The model under review builds one solid part; all positions refer to its coordinate system, in mm. A direction names the side the tool comes from. Give positions to 0.01 mm unless a question says otherwise; leave off trailing zeros. Loops run counter-clockwise (first coordinate to the right, second up) from the corner with the lowest first, then second, coordinate; pieces in that order, holes last. Notation, with made-up numbers: M -23,34.25 L 12,34.25 A17 ccw 12,54.25 Z; hole C 28,-20.5 d5. An arc over 180 degrees is marked long. One line per item, written item: value. Start each with the question number.
Q1. For pin 1 (1.7 mm diameter, centred on x = -19, z = 5, fed in from +Y); pin 2 (12 mm diameter, centred on x = 0, y = 0, fed in from -Z); pin 3 (0.8 mm diameter, centred on x = -19, z = 7.5, fed in from +Y); pin 4 (5 mm diameter, centred on x = 0, y = 0, fed in from +Z), all flat-tipped, find the tip position at first contact; note any pin that passes through.
Q2. We need section A-A on z = 5. Give the number of separate pieces and of enclosed holes in the cut face, plus the area to 3 significant figures.
Q3. Mouldability with a two-part tool opening along Y and no side actions: class faces 6 (the face through (-15, 19, 10)), 7 (the face through (-23.4, 23.43, -2.46)), 8 (the face through (14.6, -9.05, 4.93)), 9 (the face through (-19, 16, 5)) as released by +Y, released by -Y, zero draft, split by the parting line, or undercut.
Q4. We need section B-B on x = 0. Write out the cut boundary in (y, z), plus the area to 3 significant figures.
Q5. We need section D-D on z = -2.25. Write out the cut boundary in (x, y), plus the area to 3 significant figures.
Q6. For faces 1 (the face through (14, -19, 10)), 2 (the face through (19, 13, 5)), 3 (the face through (14.6, 19.95, 4.93)), 4 (the face through (23.4, -23.43, -2.46)), 5 (the face through (14.43, -10.55, 4.93)), list the 3-axis set-ups (+Z, -Z, +X, -X, +Y, -Y) from which the entire face can be reached by the end or side of a thin tool; tool diameter is ignored.
Q7. To check wall thickness, follow line 1 along Y through (x, z) = (-13, 1.25); line 2 along X through (y, z) = (18, 2); line 3 along Y through (x, z) = (13.5, 7.5). State the ranges of each line that lie inside material, in increasing order. Write a range as from..to.
```python
from build123d import *

# Parameters (mm, degrees)
F0_W           = 36
F0_H           = 36
F1_DEPTH       = 4
F3_DEPTH       = 10
F5_D           = 8
F5_CSINK_D     = 15
F5_CSINK_ANGLE = 90
F6_DEPTH       = 1


with BuildPart() as f1:
    # F0 (on Top) → F1 (new body)
    with BuildSketch(Plane.XY):
        with BuildLine():
            ThreePointArc((24, 22), (23.4142135624, 23.4142135624), (22, 24))
            Line((22, 24), (-22, 24))
            ThreePointArc((-22, 24), (-23.4142135624, 23.4142135624), (-24, 22))
            Line((-24, 22), (-24, -22))
            ThreePointArc((-24, -22), (-23.4142135624, -23.4142135624), (-22, -24))
            Line((-22, -24), (22, -24))
            ThreePointArc((22, -24), (23.4142135624, -23.4142135624), (24, -22))
            Line((24, -22), (24, 22))
        make_face()
        Rectangle(F0_W, F0_H, mode=Mode.SUBTRACT)
        Rectangle(F0_W, F0_H)
    extrude(amount=-F1_DEPTH)

    # F2 (on face) → F3 (join)
    with BuildSketch(Plane.XY):
        with BuildLine():
            Line((18.1541072781, 16), (19.7395133362, 16))
            ThreePointArc((19.7395133362, 16), (14.5, 19.95), (9.2604866638, 16))
            Line((9.2604866638, 16), (10.8458927219, 16))
            ThreePointArc((10.8458927219, 16), (14.5, 18.45), (18.1541072781, 16))
        make_face()
        with BuildLine():
            ThreePointArc((9.2604866638, 13), (14.5, 9.05), (19.7395133362, 13))
            Line((19.7395133362, 13), (18.1541072781, 13))
            ThreePointArc((18.1541072781, 13), (14.5, 10.55), (10.8458927219, 13))
            Line((10.8458927219, 13), (9.2604866638, 13))
        make_face()
        with BuildLine():
            Line((-10.8458927219, 16), (-9.2604866638, 16))
            ThreePointArc((-9.2604866638, 16), (-14.5, 19.95), (-19.7395133362, 16))
            Line((-19.7395133362, 16), (-18.1541072781, 16))
            ThreePointArc((-18.1541072781, 16), (-14.5, 18.45), (-10.8458927219, 16))
        make_face()
        with BuildLine():
            ThreePointArc((-19.7395133362, 13), (-14.5, 9.05), (-9.2604866638, 13))
            Line((-9.2604866638, 13), (-10.8458927219, 13))
            ThreePointArc((-10.8458927219, 13), (-14.5, 10.55), (-18.1541072781, 13))
            Line((-18.1541072781, 13), (-19.7395133362, 13))
        make_face()
        with BuildLine():
            Line((18.1541072781, -13), (19.7395133362, -13))
            ThreePointArc((19.7395133362, -13), (14.5, -9.05), (9.2604866638, -13))
            Line((9.2604866638, -13), (10.8458927219, -13))
            ThreePointArc((10.8458927219, -13), (14.5, -10.55), (18.1541072781, -13))
        make_face()
        with BuildLine():
            ThreePointArc((9.2604866638, -16), (14.5, -19.95), (19.7395133362, -16))
            Line((19.7395133362, -16), (18.1541072781, -16))
            ThreePointArc((18.1541072781, -16), (14.5, -18.45), (10.8458927219, -16))
            Line((10.8458927219, -16), (9.2604866638, -16))
        make_face()
        with BuildLine():
            ThreePointArc((-9.2604866638, -13), (-14.5, -9.05), (-19.7395133362, -13))
            Line((-19.7395133362, -13), (-18.1541072781, -13))
            ThreePointArc((-18.1541072781, -13), (-14.5, -10.55), (-10.8458927219, -13))
            Line((-10.8458927219, -13), (-9.2604866638, -13))
        make_face()
        with BuildLine():
            Line((-18.1541072781, -16), (-19.7395133362, -16))
            ThreePointArc((-19.7395133362, -16), (-14.5, -19.95), (-9.2604866638, -16))
            Line((-9.2604866638, -16), (-10.8458927219, -16))
            ThreePointArc((-10.8458927219, -16), (-14.5, -18.45), (-18.1541072781, -16))
        make_face()
    extrude(amount=F3_DEPTH)

    # F5 (through all)
    with Locations(Plane(origin=(0, 0, -4), x_dir=(1, 0, 0), z_dir=(0, 0, -1))):
        with Locations((0, 0)):
            CounterSinkHole(F5_D / 2, F5_CSINK_D / 2, counter_sink_angle=F5_CSINK_ANGLE)

    # F6 (add): a face of the model
    f6_faces = [f1.faces().sort_by_distance(p)[0] for p in [
        (22.9342135624, 22.9342135624, -4),
    ]]
    extrude(f6_faces, amount=F6_DEPTH)


solid = f1.part
```
Solved:
1. pin 1: y = 18.55
1. pin 2: z = -2.5
1. pin 3: y = 18.09
1. pin 4: through
2. separate pieces: 8
2. enclosed holes: 0
2. area: 141 mm2
3. face 6: zero draft
3. face 7: released by +Y
3. face 8: undercut
3. face 9: undercut
4. outline: M -24,-5 L -7.5,-5 L -7.5,-4 L -4,-0.5 L -4,0 L -24,0 Z; M 4,-0.5 L 7.5,-4 L 7.5,-5 L 24,-5 L 24,0 L 4,0 Z
4. area: 181 mm2
5. outline: M -24,-22 A2 ccw -22,-24 L 22,-24 A2 ccw 24,-22 L 24,22 A2 ccw 22,24 L -22,24 A2 ccw -24,22 Z; hole C 0,0 d11.5
5. area: 2,200 mm2
6. face 1: +Z, +X, -X, +Y, -Y
6. face 2: +Z, +X, -X
6. face 3: +Z, +Y
6. face 4: +Z, -Z, +X, -Y
6. face 5: +Z
7. line 1: -19.74..-18.15, -10.85..-9.26, 9.26..10.85, 18.15..19.74
7. line 2: -18.68..-16.33, -12.67..-10.32, 10.32..12.67, 16.33..18.68
7. line 3: -19.86..-18.32, -10.68..-9.14, 9.14..10.68, 18.32..19.86
